Check sheet for the modelled part. Datum: model origin and axes. Units: mm. Round coordinates to 2 decimals unless told otherwise and drop trailing zeros. Order: outer loops, then holes, each group sorted by start corner. A loop starts at its lowest first (then second) coordinate and runs counter-clockwise, first axis right, second up. Notation, with made-up numbers: (-16, 34) -> (29, 34) arc R18 cw to (29, 47) -> close; hole circle Ø9 at (69.5, 79). An arc over 180 degrees is marked (long way). Answer as CSV lines item,"result". Start each with the question number.
Autodesk Inventor part; units mm, degrees
ref_plane "YZ Plane" through (0, 0, 0) normal (1, 0, 0) x (0, 1, 0)
ref_plane "XZ Plane" through (0, 0, 0) normal (0, 1, 0) x (-1, 0, 0)
ref_plane "XY Plane" through (0, 0, 0) normal (0, 0, 1) x (1, 0, 0)
sketch "Sketch4" plane through (0, 0, 0) normal (0, 0, 1) x (1, 0, 0)
  line L0 (-2.4, 0) -> (10, 0)
  line L1 (0, 0) -> (-2.4, 0)
  line L2 (0, 2.8) -> (0, 1.97)
  line L3 (0.5, 1.47) -> (0.5, 1.47)
  line L4 (0.5, 1.47) -> (1, 1.5)
  arc A0 (0, 1.97) -> (0.5, 1.47) centre (0.5, 1.97) ccw
  line L5 (-2.4, 0) -> (-2.4, 1.5)
  line L6 (0, 2.8) -> (-1.4761, 2.8)
  arc A1 (-1.4761, 2.8) -> (-2.4, 1.5) centre (2.0854, -0.7093) ccw
  line L7 (1, 1.5) -> (10, 1.5)
  line L8 (10, 1.5) -> (10, 0)
  point P0 (0, 1.47)
  dimension "d71" = 0.5
  dimension "d72" = 10
  dimension "d74" = 0.5
  dimension "d75" = 2.94
  dimension "d78" = 3
  dimension "d82" = 5
  dimension "d83" = 2.4
  dimension "d84" = 5.6
  dimension "d104" = 9
  dimension "d105" = 3
revolve "Revolution7" add sketch "Sketch4" angle 360 about axis through (-2.4, 0, 0) along (1, 0, 0)
sketch "Sketch5" plane through (-2.4, 0, 0) normal (-1, 0, 0) x (0, 0, 1)
  circle A0 centre (0, 0) radius 1.4 construction
  circle A1 centre (0, 0) radius 0.98 construction
  line L0 (0, 0) -> (-0.8487, 0.49)
  line L1 (0, 0) -> (-0.8487, -0.49)
  line L2 (-1.8008, 0) -> (1.7887, 0)
  line L3 (-1.4, 0) -> (-0.8487, -0.49)
  line L4 (-1.4, 0) -> (-0.8487, 0.49)
  point P0 (0, 0)
  dimension "d88" = 2.8
  dimension "d89" = 1.96
  dimension "d90" = 30
  dimension "d91" = 30
extrude "Extrusion1" cut sketch "Sketch5" against normal blind 1.27
pattern_circular "Circular Pattern1" count 6 over 360 about axis through (-10, 0, 0) along (1, 0, 0) of "Extrusion1"
fillet "Fillet1" radius 0.28 12 edges at (-1.765, -1.2124, -0.7) (-1.765, -0.49, -0.8487) (-1.765, -0.98, 0) (-1.765, -1.2124, 0.7) (-1.765, -0.49, 0.8487) (-1.765, 0, 1.4) (-1.765, 0.98, 0) (-1.765, 1.2124, 0.7) (-1.765, 0.49, 0.8487) (-1.765, 0.49, -0.8487) (-1.765, 0, -1.4) (-1.765, 1.2124, -0.7)
thread "Thread7"
equation "\"a\" = 1"
equation "\"b\" = 9"
equation "\"dk\" = 5.6"
equation "\"k\" = 2.4"
equation "\"r\" = 0.5"
equation "\"rf\" = 5"
equation "\"x\" = 0.5"
equation "\"A_\" = 2.8"
equation "\"t\" = 1.27"
equation "\"p\" = 0.5"
equation "\"d\" = 3"
equation "\"ds_\" = 2.94"
equation "\"lg\" = 0"
properties part number "Винты со звездообразным углублением в плоско-выпуклой головке ISO 14583 — M3 x 10 — 4.8" material "Сталь"
1) Mould release check, pull along Z, two halves, no side actions. Record for faces 1 (the face through (10, 0, 0)), 2 (the face through (-1.13, 0, 0)), 3 (the face through (-0.7, -2.8, -0.1)): released by +Z, released by -Z, zero draft, split by the parting line, or undercut.
2) Depth check by flat-ended pin: pin 1 Ø2 at (x, y) = (6, 1) entering from -Z; pin 2 Ø1 at (x, z) = (6.5, -1) entering from -Y; pin 3 Ø0.7 at (y, z) = (0.5, 0) entering from -X. Enter the tip coordinate at first touch or a pass-through.
3) Material ranges on line 1 along Z through (x, y) = (-2, -0.1); line 2 along Z through (x, y) = (6.5, 0.1); line 3 along X through (y, z) = (-0.2, 0.8), recorded low to high.
4) Section check A-A on x = 3. Record the cut outline in (y, z), then the cut area to 3 significant figures.
Solutions:
1,face 1,"zero draft"
1,face 2,"undercut"
1,face 3,"split by the parting line"
2,pin 1,"stops at z = -1.5"
2,pin 2,"stops at y = -1.41"
2,pin 3,"stops at x = -1.13"
3,line 1,"z = -2.17 to -1.24, 1.24 to 2.17"
3,line 2,"z = -1.5 to 1.5"
3,line 3,"x = -1.13 to 10"
4,outline,"circle Ø3 at (0, 0)"
4,area,"7.07 mm^2"
